from build123d import *

# Parameters (mm, degrees)
F0_W     = 418
F0_H     = 50
F1_DEPTH = 15
F2_W     = 10
F2_H     = 10
F3_DEPTH = 16
F4_W     = 10
F4_H     = 10
F5_DEPTH = 16
F6_W     = 15
F6_H     = 30
F7_DEPTH = 6


# Not quite as in the source:
# - a feature names something its author has since deleted; it is built from what else it names


with BuildPart() as f1:
    # F0 (on Front) → F1 (new body)
    with BuildSketch(Plane.XZ):
        Rectangle(F0_W, F0_H)
    extrude(amount=F1_DEPTH)

    # F2 (on face) → F3 (join)
    with BuildSketch(Plane.YZ.offset(209)):
        with Locations((-7, 10)):
            Rectangle(F2_W, F2_H)
        with Locations((-7, -10)):
            Rectangle(F2_W, F2_H)
    extrude(amount=F3_DEPTH)

    # F4 (on face) → F5 (join)
    with BuildSketch(Plane(origin=(-209, 0, 0), x_dir=(0, -1, 0), z_dir=(-1, 0, 0))):
        with Locations((7, 10)):
            Rectangle(F4_W, F4_H)
        with Locations((7, -10)):
            Rectangle(F4_W, F4_H)
    extrude(amount=F5_DEPTH)

    # F6 (on face) → F7 (cut)
    with BuildSketch(Plane.XZ):
        with Locations((51.5, 10)):
            Rectangle(F6_W, F6_H)
    extrude(amount=F7_DEPTH, mode=Mode.SUBTRACT)


solid = f1.part
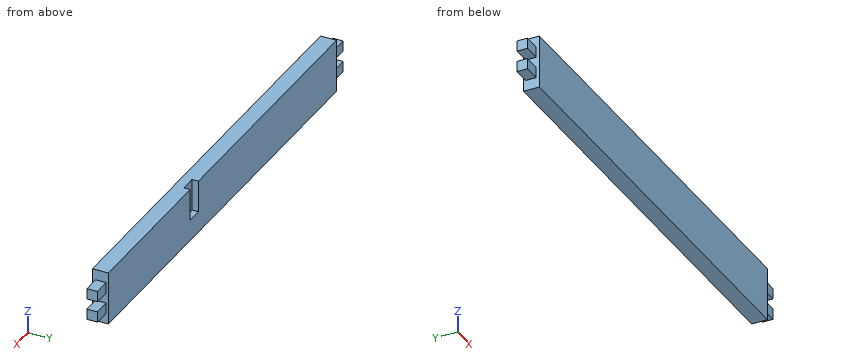
For this review, take the finished solid that the model builds, in its own axes (mm). Coordinates: 2 decimals unless noted, no trailing zeros. Loops run counter-clockwise (first coordinate to the right, second up) from the corner with the lowest first, then second, coordinate; pieces in that order, holes last. Notation, with made-up numbers: (89.5, 49.25) - (114.5, 49.25) arc R24 ccw to (114.5, 69.25) - close; hole circle Ø6 at (25, -11.5). An arc over 180 degrees is marked (long way). Use a Markdown table: item, result. Add a question column.
Item 1: We need section B-B (y = -8.25). Give the boundary of the cut face in (x, z).
Item 2: For line 1 (X direction, y = -4, z = 22); line 2 (X direction, y = -12.75, z = 6), list the stretches that pass through material, from the lowest coordinate up.
Item 3: We need section C-C (z = 21). Give the boundary of the cut face in (x, y).
Item 4: We need section A-A (z = -10). Give the boundary of the cut face in (x, y).
Item 5: Insertion check: pin 1 Ø11 at (x, z) = (213, -12.5) entering from +Y; pin 2 Ø8 at (x, y) = (-215, -7) entering from -Z; pin 3 Ø8 at (x, z) = (216.5, -9.5) entering from -Y; pin 4 Ø3 at (x, z) = (218, 12.5) entering from +Y. Each pin has a flat end and moves straight along its axis. Give the tip position at first contact, or say it passes through.
Results list:
| question | item | result |
|---|---|---|
| 1 | outline | (-225, -15) - (-209, -15) - (-209, -25) - (209, -25) - (209, -15) - (225, -15) - (225, -5) - (209, -5) - (209, 5) - (225, 5) - (225, 15) - (209, 15) - (209, 25) - (-209, 25) - (-209, 15) - (-225, 15) - (-225, 5) - (-209, 5) - (-209, -5) - (-225, -5) - close |
| 2 | line 1 | x = -209 to 44, 59 to 209 |
| 2 | line 2 | x = -209 to 209 |
| 3 | outline | (-209, -15) - (209, -15) - (209, 0) - (59, 0) - (59, -6) - (44, -6) - (44, 0) - (-209, 0) - close |
| 4 | outline | (-225, -12) - (-209, -12) - (-209, -15) - (209, -15) - (209, -12) - (225, -12) - (225, -2) - (209, -2) - (209, 0) - (-209, 0) - (-209, -2) - (-225, -2) - close |
| 5 | pin 1 | stops at y = 0 |
| 5 | pin 2 | stops at z = -15 |
| 5 | pin 3 | stops at y = -12 |
| 5 | pin 4 | stops at y = -2 |
